Check sheet for the modelled part. Datum: model origin and axes. Units: mm. A direction names the side the tool comes from. Round coordinates to 2 decimals unless told otherwise and drop trailing zeros. Write each loop counter-clockwise with the first axis right and the second up, starting at its lowest first coordinate (ties: lowest second). Pieces come first, ordered by that corner, then holes. Notation, with made-up numbers: (74, 21) -> (86, 21) arc R33 ccw to (86, 57) -> close; hole circle Ø10 at (19, -12). An arc over 180 degrees is marked (long way). Put each result on its own line as item: value. Start each with the question number.
from build123d import *

# Parameters (mm, degrees)
SKETCH_R        = 4.3
PAD_DEPTH       = 10
SKETCH001_R     = 3.3
POCKET_DEPTH    = 10.001
POCKET001_DEPTH = 5.2
FILLET_R        = 3
SKETCH003_W     = 26
SKETCH003_H     = 70
POCKET002_DEPTH = 5


with BuildPart() as part:
    # Sketch → Pad (new body)
    with BuildSketch(Plane.XY):
        Polygon((76, 0), (76, 67), (50, 68.5), (26, 68.5), (0, 67), (0, 0), (26, -1.5), (50, -1.5), align=None)
        with Locations((11, 58.5)):
            Circle(SKETCH_R, mode=Mode.SUBTRACT)
        with Locations((65, 58.5)):
            Circle(SKETCH_R, mode=Mode.SUBTRACT)
        with Locations((65, 8.5)):
            Circle(SKETCH_R, mode=Mode.SUBTRACT)
        with Locations((11, 8.5)):
            Circle(SKETCH_R, mode=Mode.SUBTRACT)
    extrude(amount=PAD_DEPTH)

    # Sketch001 (on Face14 of Pad) → Pocket (cut, through all)
    with BuildSketch(Plane.XY.offset(10)):
        with Locations((38, 61.5)):
            Circle(SKETCH001_R)
        with Locations((38, 5.5)):
            Circle(SKETCH001_R)
    extrude(amount=-POCKET_DEPTH, mode=Mode.SUBTRACT)

    # Sketch002 (on Face4 of Pocket) → Pocket001 (cut)
    with BuildSketch(Plane(origin=(0, 0, 0), x_dir=(1, 0, 0), z_dir=(0, 0, -1))):
        Polygon((40.973354, -10.65), (43.946708, -5.5), (40.973354, -0.35), (35.026646, -0.35), (32.053292, -5.5), (35.026646, -10.65), align=None)
        Polygon((43.946708, -61.5), (40.973354, -56.35), (35.026646, -56.35), (32.053292, -61.5), (35.026646, -66.65), (40.973354, -66.65), align=None)
    extrude(amount=-POCKET001_DEPTH, mode=Mode.SUBTRACT)

    # Fillet
    fillet_edges = [part.edges().sort_by_distance(p)[0] for p in [
        (0, 67, 5),
        (0, 0, 5),
        (76, 0, 5),
        (76, 67, 5),
    ]]
    fillet(fillet_edges, radius=FILLET_R)

    # Sketch003 (on Face5 of Fillet) → Pocket002 (cut)
    with BuildSketch(Plane.XY.offset(10)):
        with Locations((13, 33.5)):
            Rectangle(SKETCH003_W, SKETCH003_H)
    extrude(amount=-POCKET002_DEPTH, mode=Mode.SUBTRACT)


solid = part.part
1. Draft check along X on faces 4 (the flat face through (37, 34, 0)), 5 (the flat face through (26, 33, 8)), 6 (the flat face through (33.56, 2.89, 2.56)). Enter one of: released by +X, released by -X, zero draft, split by the parting line, or undercut.
2. Section check D-D, the plane x = 12. Enter the section's corners in (y, z).
3. Material ranges on L1, parallel to Y at x = 38, z = 8.2; L2, parallel to Y at x = 39, z = 2.75; L3, parallel to X at y = 47, z = 6, recorded low to high. Write a range as [from, to].
4. Section check C-C, the plane z = 7.5. Enter the section's corners in (x, y).
5. Gauge pin test, flat ends, axial feed: P1, Ø7, axis at x = 11, y = 58.5, coming from the +Z side; P2, Ø8, axis at x = 8.5, y = 46.5, coming from the +Z side; P3, Ø3, axis at x = 36, y = 63.5, coming from the -Z side; P4, Ø1.5, axis at y = 20, z = 8.5, coming from the -X side. Record the tip position at first contact, or that the pin passes through.
6. Section check A-A, the plane x = 38. Enter the section's corners in (y, z), then the cut area to 3 significant figures.
7. Section check B-B, the plane z = 2.75. Enter the section's corners in (x, y).
8. Access from +Z, -Z, +X, -X, +Y, -Y to the whole of each face (thin tool, end or side, straight path). Record for faces 1 (the cylindrical face through (0.84, 66.25, 2.54)), 2 (the flat face through (13, 34, 5)), 3 (the flat face through (33.56, 58.89, 2.56)).
Reply:
1. face 4: zero draft
1. face 5: released by -X
1. face 6: undercut
2. outline: (-0.69, 0) -> (4.32, 0) -> (4.32, 5) -> (-0.69, 5) -> close; (12.68, 0) -> (54.32, 0) -> (54.32, 5) -> (12.68, 5) -> close; (62.68, 0) -> (67.69, 0) -> (67.69, 5) -> (62.68, 5) -> close
3. L1: y = [-1.5, 2.2], [8.8, 58.2], [64.8, 68.5]
3. L2: y = [-1.5, 0.35], [10.65, 56.35], [66.65, 68.5]
3. L3: x = [26, 76]
4. outline: (26, -1.5) -> (50, -1.5) -> (73.17, -0.16) arc R3 ccw to (76, 2.83) -> (76, 64.17) arc R3 ccw to (73.17, 67.16) -> (50, 68.5) -> (26, 68.5) -> close; hole circle Ø6.6 at (38, 5.5); hole circle Ø6.6 at (38, 61.5); hole circle Ø8.6 at (65, 8.5); hole circle Ø8.6 at (65, 58.5)
5. P1: passes through
5. P2: stops at z = 5
5. P3: stops at z = 5.2
5. P4: stops at x = 26
6. outline: (-1.5, 0) -> (0.35, 0) -> (0.35, 5.2) -> (2.2, 5.2) -> (2.2, 10) -> (-1.5, 10) -> close; (8.8, 5.2) -> (10.65, 5.2) -> (10.65, 0) -> (56.35, 0) -> (56.35, 5.2) -> (58.2, 5.2) -> (58.2, 10) -> (8.8, 10) -> close; (64.8, 5.2) -> (66.65, 5.2) -> (66.65, 0) -> (68.5, 0) -> (68.5, 10) -> (64.8, 10) -> close
6. area: 530 mm2
7. outline: (0, 2.83) arc R3 ccw to (2.83, -0.16) -> (26, -1.5) -> (50, -1.5) -> (73.17, -0.16) arc R3 ccw to (76, 2.83) -> (76, 64.17) arc R3 ccw to (73.17, 67.16) -> (50, 68.5) -> (26, 68.5) -> (2.83, 67.16) arc R3 ccw to (0, 64.17) -> close; hole circle Ø8.6 at (11, 8.5); hole circle Ø8.6 at (11, 58.5); hole (32.05, 5.5) -> (35.03, 0.35) -> (40.97, 0.35) -> (43.95, 5.5) -> (40.97, 10.65) -> (35.03, 10.65) -> close; hole (32.05, 61.5) -> (35.03, 56.35) -> (40.97, 56.35) -> (43.95, 61.5) -> (40.97, 66.65) -> (35.03, 66.65) -> close; hole circle Ø8.6 at (65, 8.5); hole circle Ø8.6 at (65, 58.5)
8. face 1: +Z, -Z, -X, +Y
8. face 2: +Z, -X, +Y, -Y
8. face 3: -Z
